The model under review builds one solid part; all positions refer to its coordinate system, in mm. Face numbers are marked on the shaded views. Coordinates: 2 decimals unless noted, no trailing zeros. Write each loop counter-clockwise with the first axis right and the second up, starting at its lowest first coordinate (ties: lowest second). Pieces come first, ordered by that corner, then holes. Notation, with made-up numbers: (69, 45.25) - (103, 45.25) arc R18 cw to (103, 77.25) - close; hole circle Ø6 at (55.5, 41.5). An arc over 180 degrees is marked (long way). Return JSON: item names as keys, results as strings. Group by question number.
(1) Draft analysis for pull direction Y (two halves, no side actions). For the marked faces 1, 2 and 3, state which applies: released by +Y, released by -Y, zero draft, split by the parting line, or undercut.
(2) We need section C-C on x = 0. State the section outline as (y, z) points, then the cut area to 3 significant figures.
(3) To check wall thickness, follow L1, parallel to Y at x = -2, z = 0; L2, parallel to Y at x = 0, z = 2; L3, parallel to Z at x = 2.5, y = 3. State the ranges of each line that lie inside material, in increasing order. Write a range as from..to.
(4) We need section B-B on y = 7. State the section outline as (x, z) points, then the cut area to 3 significant figures.
(5) For pin 1 Ø1 at (x, z) = (1, -1.5) entering from -Y; pin 2 Ø2 at (y, z) = (3.048, 0) entering from +X (3 decimals), all flat-tipped, find the tip position at first contact; note any pin that passes through.
(6) We need section D-D on x = 1.5. State the section outline as (y, z) points, then the cut area to 3 significant figures.
(7) We need section A-A on z = 0.25. State the section outline as (x, y) points.
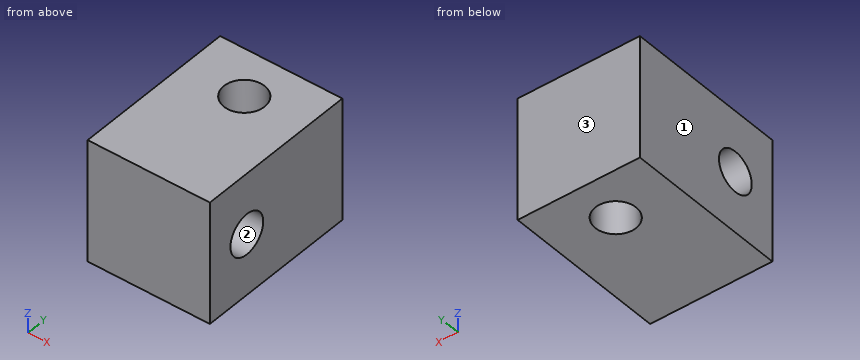
```python
from build123d import *

# Parameters (mm, degrees)
SKETCH1_W                  = 10.922
SKETCH1_H                  = 8.128
BOSS_EXTRUDE1_DEPTH        = 8.128
M2_5_CLEARANCE_HOLE1_D     = 2.7051
M2_5_CLEARANCE_HOLE1_DEPTH = 8.128
M2_5_CLEARANCE_HOLE2_D     = 2.7051
M2_5_CLEARANCE_HOLE2_DEPTH = 8.128


with BuildPart() as part:
    # Sketch1 → Boss-Extrude1 (new body)
    with BuildSketch(Plane(origin=(-4.064, 0, 0), x_dir=(0, -1, 0), z_dir=(-1, 0, 0))):
        with Locations((-5.461, 0)):
            Rectangle(SKETCH1_W, SKETCH1_H)
    extrude(amount=-BOSS_EXTRUDE1_DEPTH)

    # M2.5 Clearance Hole1
    with Locations(Plane(origin=(4.064, 0, 0), x_dir=(0, 0, -1), z_dir=(1, 0, 0))):
        with Locations((0, 3.048)):
            Hole(M2_5_CLEARANCE_HOLE1_D / 2, depth=M2_5_CLEARANCE_HOLE1_DEPTH)

    # M2.5 Clearance Hole2
    with Locations(Plane.XY.offset(4.064)):
        with Locations((0, 7.874)):
            Hole(M2_5_CLEARANCE_HOLE2_D / 2, depth=M2_5_CLEARANCE_HOLE2_DEPTH)


solid = part.part
```
Ans:
{
 "1": {"face 1": "zero draft", "face 2": "undercut", "face 3": "released by +Y"},
 "2": {"outline": "(0, -4.06) - (6.52, -4.06) - (6.52, 4.06) - (0, 4.06) - close; (9.23, -4.06) - (10.92, -4.06) - (10.92, 4.06) - (9.23, 4.06) - close; hole circle Ø2.71 at (3.05, 0)", "area": "61.0 mm²"},
 "3": {"L1": "0..1.7, 4.4..10.92", "L2": "0..6.52, 9.23..10.92", "L3": "-4.06..-1.35, 1.35..4.06"},
 "4": {"outline": "(-4.06, -4.06) - (-1.03, -4.06) - (-1.03, 4.06) - (-4.06, 4.06) - close; (1.03, -4.06) - (4.06, -4.06) - (4.06, 4.06) - (1.03, 4.06) - close", "area": "49.3 mm²"},
 "5": {"pin 1": "y = 0", "pin 2": "through"},
 "6": {"outline": "(0, -4.06) - (10.92, -4.06) - (10.92, 4.06) - (0, 4.06) - close; hole circle Ø2.71 at (3.05, 0)", "area": "83.0 mm²"},
 "7": {"outline": "(-4.06, 0) - (4.06, 0) - (4.06, 1.72) - (-4.06, 1.72) - close; (-4.06, 4.38) - (4.06, 4.38) - (4.06, 10.92) - (-4.06, 10.92) - close; hole circle Ø2.71 at (0, 7.87)"}
}
